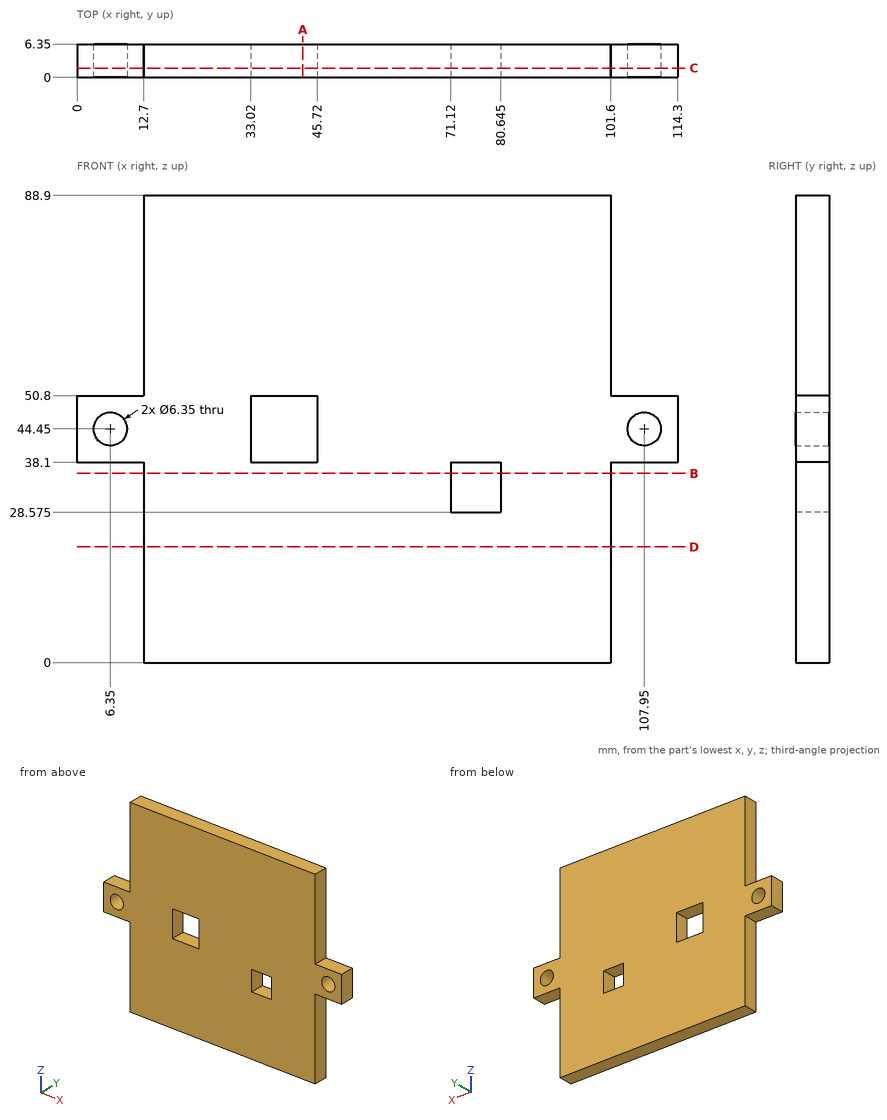
Print and shaded views of the part. All mm, measured from the part's lowest x, y and z. Coordinates: 2 decimals unless noted, no trailing zeros. Write each loop counter-clockwise with the first axis right and the second up, starting at its lowest first coordinate (ties: lowest second). Pieces come first, ordered by that corner, then holes. Notation, with made-up numbers: M 48,3 L 96,3 A34 cw 96,39 Z; hole C 36.5,4.25 d5. An arc over 180 degrees is marked long. Return JSON: item names as keys, results as strings.
1. Probe L1, parallel to Z at x = 107.95, y = 2 (3 decimals); L2, parallel to Z at x = 35, y = 5.5; L3, parallel to X at y = 1.25, z = 60. List the from-to ranges inside material, lowest first.
Determined:
{"L1": "38.1 to 41.275, 47.625 to 50.8", "L2": "0 to 38.1, 50.8 to 88.9", "L3": "12.7 to 101.6"}
2. Flat gauge pins, fed straight in: pin 1 Ø3 at (x, y) = (3.5, 2) entering from -Z; pin 2 Ø3 at (y, z) = (3, 64.5) entering from +X; pin 3 Ø3 at (x, y) = (3.5, 3) entering from +Z. Where does each tip first touch, or does it go through?
Determined:
{"pin 1": "z = 38.1", "pin 2": "x = 101.6", "pin 3": "z = 50.8"}
3. Saw through at C-C, the plane y = 1.75. Write the cut outline in (x, z) (3 decimals).
Determined:
{"outline": "M 0,38.1 L 12.7,38.1 L 12.7,0 L 101.6,0 L 101.6,38.1 L 114.3,38.1 L 114.3,50.8 L 101.6,50.8 L 101.6,88.9 L 12.7,88.9 L 12.7,50.8 L 0,50.8 Z; hole C 6.35,44.45 d6.35; hole M 33.02,38.1 L 45.72,38.1 L 45.72,50.8 L 33.02,50.8 Z; hole M 71.12,28.575 L 80.645,28.575 L 80.645,38.1 L 71.12,38.1 Z; hole C 107.95,44.45 d6.35"}
4. Saw through at B-B, the plane z = 36. Write the cut outline in (x, y) (3 decimals), then the cut area to 3 significant figures.
Determined:
{"outline": "M 12.7,0 L 71.12,0 L 71.12,6.35 L 12.7,6.35 Z; M 80.645,0 L 101.6,0 L 101.6,6.35 L 80.645,6.35 Z", "area": "504 mm²"}
5. Saw through at A-A, the plane x = 43. Write the cut outline in (y, z).
Determined:
{"outline": "M 0,0 L 6.35,0 L 6.35,38.1 L 0,38.1 Z; M 0,50.8 L 6.35,50.8 L 6.35,88.9 L 0,88.9 Z"}
6. Saw through at D-D, the plane z = 22. Write the cut outline in (x, y), then the cut area to 3 significant figures.
Determined:
{"outline": "M 12.7,0 L 101.6,0 L 101.6,6.35 L 12.7,6.35 Z", "area": "565 mm²"}
